Could you check a few things on this model? Use its own coordinates, in mm. A direction names the side the tool comes from. Give positions to 0.01 mm unless a question says otherwise; leave off trailing zeros. Order: outer loops, then holes, each group sorted by start corner. A loop starts at its lowest first (then second) coordinate and runs counter-clockwise, first axis right, second up.
from build123d import *

# Parameters (mm, degrees)
SKETCH1_W           = 40
SKETCH1_H           = 55
BOSS_EXTRUDE1_DEPTH = 25
SKETCH2_W           = 35.5
SKETCH2_H           = 21
CUT_EXTRUDE1_DEPTH  = 52.5
SKETCH3_R           = 1.485145447
CUT_EXTRUDE2_DEPTH  = 52.5
SKETCH5_W           = 33.510072246
SKETCH5_H           = 13.913042654
CUT_EXTRUDE3_DEPTH  = 20


with BuildPart() as part:
    # Sketch1 → Boss-Extrude1 (new body)
    with BuildSketch(Plane(origin=(0, 0, 0), x_dir=(1, 0, 0), z_dir=(0, 1, 0))):
        Rectangle(SKETCH1_W, SKETCH1_H)
    extrude(amount=BOSS_EXTRUDE1_DEPTH)

    # Sketch2 → Cut-Extrude1 (cut)
    with BuildSketch(Plane.XY.offset(27.5)):
        with Locations((0.05, 12.1)):
            Rectangle(SKETCH2_W, SKETCH2_H)
    extrude(amount=-CUT_EXTRUDE1_DEPTH, mode=Mode.SUBTRACT)

    # Sketch3 → Cut-Extrude2 (cut)
    with BuildSketch(Plane.ZY.offset(20)):
        with Locations((23.566951269, 12.5)):
            Circle(SKETCH3_R)
    extrude(amount=-CUT_EXTRUDE2_DEPTH, mode=Mode.SUBTRACT)

    # Sketch5 → Cut-Extrude3 (cut)
    with BuildSketch(Plane(origin=(0, 25, 0), x_dir=(1, 0, 0), z_dir=(0, 1, 0))):
        with Locations((0, -17.264049878)):
            Rectangle(SKETCH5_W, SKETCH5_H)
    extrude(amount=-CUT_EXTRUDE3_DEPTH, mode=Mode.SUBTRACT)


solid = part.part
Item 1: We'd pull the mould along Y, two halves only. Please class faces 4 (the flat face through (20, 12, 0)), 5 (the flat face through (0, 12, -25)), 6 (the flat face through (0, 0, 0)): +Y half, -Y half, draft (parallel to the pull), parting line (faces both ways), or undercut.
Findings:
face 4: draft
face 5: undercut
face 6: -Y half
Item 2: Imagine slicing it at A-A on y = 12.5. List the corners of the cut face in (x, z) for me.
Findings:
outline: (-20, -27.5) - (20, -27.5) - (20, 22.08) - (17.8, 22.08) - (17.8, -25) - (-17.7, -25) - (-17.7, 22.08) - (-20, 22.08) - close; (-20, 25.05) - (-17.7, 25.05) - (-17.7, 27.5) - (-20, 27.5) - close; (17.8, 25.05) - (20, 25.05) - (20, 27.5) - (17.8, 27.5) - close
Item 3: For faces 1 (the flat face through (0, 12, -27.5)), 2 (the flat face through (16.755, 24, 17)), 3 (the flat face through (0, 1.6, 2)), which set-ups out of +Z, -Z, +X, -X, +Y, -Y let a thin tool reach every point of the face, with its end or its side?
Findings:
face 1: -Z, +X, -X, +Y, -Y
face 2: +Y
face 3: +Z
Item 4: Imagine slicing it at C-C on x = -7.5. List the corners of the cut face in (y, z) for me.
Findings:
outline: (0, -27.5) - (25, -27.5) - (25, 10.31) - (22.6, 10.31) - (22.6, -25) - (1.6, -25) - (1.6, 27.5) - (0, 27.5) - close; (22.6, 24.22) - (25, 24.22) - (25, 27.5) - (22.6, 27.5) - close
Item 5: Imagine slicing it at B-B on z = -3.5. List the corners of the cut face in (x, y) for me, then the cut area to 4 significant figures.
Findings:
outline: (-20, 0) - (20, 0) - (20, 25) - (-20, 25) - close; hole (-17.7, 1.6) - (17.8, 1.6) - (17.8, 22.6) - (-17.7, 22.6) - close
area: 254.5 mm2
Item 6: For pin 1 (6 mm diameter, centred on x = 0.5, y = 10.5, fed in from +Z), with a flat end and sliding along its axis, tell me the tip position at first contact or that it passes through.
Findings:
pin 1: stops at z = -25
Item 7: Imagine slicing it at D-D on y = 19.25. List the corners of the cut face in (x, z) for me, then the cut area to 3 significant figures.
Findings:
outline: (-20, -27.5) - (20, -27.5) - (20, 27.5) - (17.8, 27.5) - (17.8, -25) - (-17.7, -25) - (-17.7, 27.5) - (-20, 27.5) - close
area: 336 mm2
Item 8: Please list where these lines run through material, in increasing order: line 1 along X through (y, z) = (7.25, 7.5); line 2 along Y through (x, z) = (6.5, -18); line 3 along Z through (x, y) = (-4.5, 4.75).
Findings:
line 1: x = -20 to -17.7, 17.8 to 20
line 2: y = 0 to 1.6, 22.6 to 25
line 3: z = -27.5 to -25
